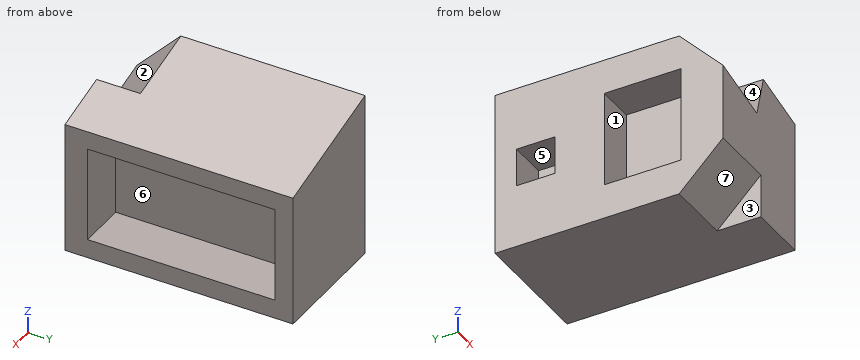
```python
from build123d import *

# Parameters (mm, degrees)
BOSS_EXTRUDE1_DEPTH = 594.610278
SKETCH3_W           = 247.65
SKETCH3_H           = 488.95
CUT_EXTRUDE1_DEPTH  = 127
SKETCH4_W           = 200
SKETCH4_H           = 250
CUT_EXTRUDE2_DEPTH  = 100
SKETCH5_W           = 100
SKETCH5_H           = 100
CUT_EXTRUDE3_DEPTH  = 100
CUT_EXTRUDE4_DEPTH  = 172
CUT_EXTRUDE5_DEPTH  = 190


with BuildPart() as part:
    # Sketch2 → Boss-Extrude1 (new body)
    with BuildSketch(Plane(origin=(0, 0, 0), x_dir=(1, 0, 0), z_dir=(0, 1, 0))):
        Polygon((0, -431.8), (327.385580216, -344.077298168), (327.385580216, 0), (0, 0), align=None)
    extrude(amount=BOSS_EXTRUDE1_DEPTH)

    # Sketch3 → Cut-Extrude1 (cut)
    with BuildSketch(Plane(origin=(327.385580216, 0, 0), x_dir=(0, 0, -1), z_dir=(1, 0, 0))):
        with Locations((-173.171445322, 303.629475409)):
            Rectangle(SKETCH3_W, SKETCH3_H)
    extrude(amount=-CUT_EXTRUDE1_DEPTH, mode=Mode.SUBTRACT)

    # Sketch4 → Cut-Extrude2 (cut)
    with BuildSketch(Plane(origin=(0, 0, 0), x_dir=(0, -1, 0), z_dir=(1, 0, 0))):
        with Locations((-209.55, -215.9)):
            Rectangle(SKETCH4_W, SKETCH4_H)
    extrude(amount=CUT_EXTRUDE2_DEPTH, mode=Mode.SUBTRACT)

    # Sketch5 → Cut-Extrude3 (cut)
    with BuildSketch(Plane.ZY):
        with Locations((215.9, 488.315)):
            Rectangle(SKETCH5_W, SKETCH5_H)
    extrude(amount=-CUT_EXTRUDE3_DEPTH, mode=Mode.SUBTRACT)

    # Sketch6 → Cut-Extrude4 (cut)
    with BuildSketch(Plane.ZY):
        Polygon((0, 114.3), (114.3, 0), (0, 0), align=None)
    extrude(amount=-CUT_EXTRUDE4_DEPTH, mode=Mode.SUBTRACT)

    # Sketch7 → Cut-Extrude5 (cut)
    with BuildSketch(Plane(origin=(-107.95, 0, 28.925115323), x_dir=(0, 1, 0), z_dir=(0.9659258262890691, 0, -0.258819045102518))):
        Polygon((0, 417.086771792), (114.3, 417.086771792), (0, 302.786771792), align=None)
    extrude(amount=CUT_EXTRUDE5_DEPTH, mode=Mode.SUBTRACT)


solid = part.part
```
Check sheet for the modelled part. Datum: model origin and axes. Units: mm. Face numbers are marked on the shaded views. A direction names the side the tool comes from. Give positions to 0.01 mm unless a question says otherwise; leave off trailing zeros. Loops run counter-clockwise (first coordinate to the right, second up) from the corner with the lowest first, then second, coordinate; pieces in that order, holes last. Notation, with made-up numbers: (-27, 23) - (-14, 23) arc R22 ccw to (-14, 36) - close; hole circle Ø4 at (-17.75, 47.5). An arc over 180 degrees is marked (long way). One line per question, with ' | ' between items. Start each with the question number.
1. Gauge pin test, flat ends, axial feed: pin 1 Ø5 at (x, y) = (178, 510.5) entering from +Z; pin 2 Ø3 at (x, y) = (61, 106.5) entering from +Z; pin 3 Ø5 at (y, z) = (189, 329.5) entering from -X; pin 4 Ø1 at (x, y) = (90, 482) entering from -Z. Record the tip position at first contact, or that the pin passes through.
2. Draft check along X on the marked faces 1, 2, 3 and 4. Enter one of: released by +X, released by -X, zero draft, split by the parting line, or undercut.
3. Set-up check for the marked faces 5, 6 and 7: record each of +Z, -Z, +X, -X, +Y, -Y from which the full face is reachable in a straight line by a thin tool's end or side.
4. Cross-section at D-D, the plane x = 49. Enter the section's corners in (y, z) (3 decimals), plus the area to 3 significant figures.
5. Cross-section at B-B, the plane x = 235. Enter the section's corners in (y, z).
6. Cross-section at A-A, the plane y = 343.5. Enter the section's corners in (x, z), plus the area to 3 significant figures.
7. Cross-section at C-C, the plane z = 77.5. Enter the section's corners in (x, y), plus the area to 3 significant figures.
8. Material ranges on line 1 along Y through (x, z) = (32.5, 184.5) (3 decimals); line 2 along Y through (x, z) = (294, 244.5); line 3 along Y through (x, z) = (49.5, 126.5), recorded low to high. Write a range as [from, to].
Check result:
1) pin 1: stops at z = 384.77 | pin 2: stops at z = 408.98 | pin 3: stops at x = 100 | pin 4: stops at z = 0
2) face 1: zero draft | face 2: undercut | face 3: released by -X | face 4: undercut
3) face 5: -X | face 6: +X | face 7: -Z, -X, -Y
4) outline: (0, 114.3) - (114.3, 0) - (594.61, 0) - (594.61, 418.67) - (114.3, 418.67) - (0, 300.338) - close; hole (109.55, 90.9) - (309.55, 90.9) - (309.55, 340.9) - (109.55, 340.9) - close; hole (438.315, 165.9) - (538.315, 165.9) - (538.315, 265.9) - (438.315, 265.9) - close | area: 176,000 mm2
5) outline: (0, 0) - (594.61, 0) - (594.61, 368.83) - (0, 368.83) - close; hole (59.15, 49.35) - (548.1, 49.35) - (548.1, 297) - (59.15, 297) - close
6) outline: (0, 0) - (327.39, 0) - (327.39, 49.35) - (200.39, 49.35) - (200.39, 297) - (327.39, 297) - (327.39, 344.08) - (0, 431.8) - close | area: 95,600 mm2
7) outline: (0, 36.8) - (172, 36.8) - (172, 0) - (327.39, 0) - (327.39, 59.15) - (200.39, 59.15) - (200.39, 548.1) - (327.39, 548.1) - (327.39, 594.61) - (0, 594.61) - close | area: 126,000 mm2
8) line 1: y = [0, 109.55], [309.55, 438.315], [538.315, 594.61] | line 2: y = [0, 59.15], [548.1, 594.61] | line 3: y = [0, 109.55], [309.55, 594.61]
